Could you check a few things on this model? Use its own coordinates, in mm. Face numbers are marked on the shaded views. A direction names the side the tool comes from. Coordinates: 2 decimals unless noted, no trailing zeros. Order: outer loops, then holes, each group sorted by start corner. A loop starts at its lowest first (then second) coordinate and runs counter-clockwise, first axis right, second up. Notation, with made-up numbers: (-16, 33) -> (13, 33) arc R9 cw to (13, 47) -> close; hole circle Ø10 at (17, 24.5). An arc over 180 degrees is marked (long way). Return JSON: item names as keys, results as strings. Group by question number.
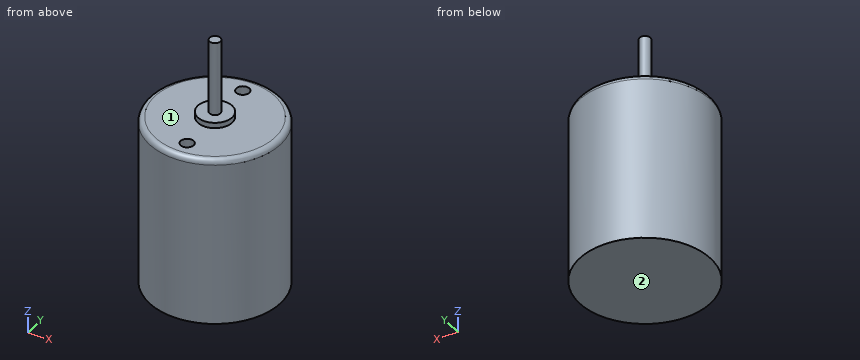
from build123d import *

# Parameters (mm, degrees)
SKETCH1_R           = 12
BOSS_EXTRUDE1_DEPTH = 31
FILLET1_R           = 1
SKETCH2_R           = 3.15
BOSS_EXTRUDE2_DEPTH = 1
SKETCH4_R           = 1
BOSS_EXTRUDE3_DEPTH = 45.6
SKETCH5_R           = 1.2
CUT_EXTRUDE1_DEPTH  = 3


with BuildPart() as part:
    # Sketch1 → Boss-Extrude1 (new body)
    with BuildSketch(Plane.XY):
        Circle(SKETCH1_R)
    extrude(amount=BOSS_EXTRUDE1_DEPTH)

    # Fillet1
    fillet1_edges = [part.edges().sort_by_distance(p)[0] for p in [
        (-12, 0, 31),
    ]]
    fillet(fillet1_edges, radius=FILLET1_R)

    # Sketch2 → Boss-Extrude2 (add)
    with BuildSketch(Plane.XY.offset(31)):
        Circle(SKETCH2_R)
    extrude(amount=BOSS_EXTRUDE2_DEPTH)

    # Sketch4 → Boss-Extrude3 (add)
    with BuildSketch(Plane(origin=(0, 0, 0), x_dir=(-1, 0, 0), z_dir=(0, 0, -1))):
        Circle(SKETCH4_R)
    extrude(amount=-BOSS_EXTRUDE3_DEPTH)

    # Sketch5 → Cut-Extrude1 (cut)
    with BuildSketch(Plane.XY.offset(31)):
        with Locations((0, -8.5)):
            Circle(SKETCH5_R)
    cut_extrude1 = extrude(amount=-CUT_EXTRUDE1_DEPTH, mode=Mode.SUBTRACT)

    # Mirror1: Cut-Extrude1 across plane
    add(cut_extrude1.mirror(Plane.ZX), mode=Mode.SUBTRACT)


solid = part.part
Q1. I'm going to push flat-ended pins straight in: pin 1 Ø1.9 at (x, y) = (0.5, 8) entering from +Z; pin 2 Ø4 at (x, z) = (2.5, 5.5) entering from -Y; pin 3 Ø5 at (y, z) = (7, 25) entering from +X. Where does each tip first touch, or does it pass through?
Q2. I want a section at C-C on z = 28.5. Please give me the cut outline in (x, y), and give its area (3 significant figures).
Q3. I need wall thicknesses on line 1 along Y through (x, z) = (0, 29.85); line 2 along Y through (x, z) = (0, 30.45); line 3 along Z through (x, y) = (0, 2). Which ranges of each line are inside material? Lowest first, please. Write a range as from..to.
Q4. I want a section at A-A on x = 0. Please give me the cut outline in (y, z), and give its area (3 significant figures).
Q5. I want a section at B-B on y = 0. Please give me the cut outline in (x, z), and give its area (3 significant figures).
Q6. I want a section at D-D on z = 40. Please give me the cut outline in (x, y), and give its area (3 significant figures).
Q7. On a 3-axis mill with a long thin cutter (end or side, diameter ignored), from which of +Z, -Z, +X, -X, +Y, -Y can I reach the whole of each face in a straight line? I mean the marked faces 1 and 2. Say none if no direction works.
Response values:
{
 "1": {"pin 1": "stops at z = 31", "pin 2": "stops at y = -11.99", "pin 3": "stops at x = 11.12"},
 "2": {"outline": "circle Ø24 at (0, 0); hole circle Ø2.4 at (0, -8.5); hole circle Ø2.4 at (0, 8.5)", "area": "443 mm²"},
 "3": {"line 1": "y = -12..-9.7, -7.3..7.3, 9.7..12", "line 2": "y = -11.89..-9.7, -7.3..7.3, 9.7..11.89", "line 3": "z = 0..32"},
 "4": {"outline": "(-12, 0) -> (12, 0) -> (12, 30) arc R1 ccw to (11, 31) -> (9.7, 31) -> (9.7, 28) -> (7.3, 28) -> (7.3, 31) -> (3.15, 31) -> (3.15, 32) -> (1, 32) -> (1, 45.6) -> (-1, 45.6) -> (-1, 32) -> (-3.15, 32) -> (-3.15, 31) -> (-7.3, 31) -> (-7.3, 28) -> (-9.7, 28) -> (-9.7, 31) -> (-11, 31) arc R1 ccw to (-12, 30) -> close", "area": "763 mm²"},
 "5": {"outline": "(-12, 0) -> (12, 0) -> (12, 30) arc R1 ccw to (11, 31) -> (3.15, 31) -> (3.15, 32) -> (1, 32) -> (1, 45.6) -> (-1, 45.6) -> (-1, 32) -> (-3.15, 32) -> (-3.15, 31) -> (-11, 31) arc R1 ccw to (-12, 30) -> close", "area": "777 mm²"},
 "6": {"outline": "circle Ø2 at (0, 0)", "area": "3.14 mm²"},
 "7": {"face 1": "+Z", "face 2": "-Z, +X, -X, +Y, -Y"}
}
